Input: dimensioned drawing with shaded views. Units: mm. Origin: part minimum x, y, z. Give positions to 0.01 mm unless a question says otherwise; leave off trailing zeros. Loops run counter-clockwise (first coordinate to the right, second up) from the corner with the lowest first, then second, coordinate; pieces in that order, holes last.
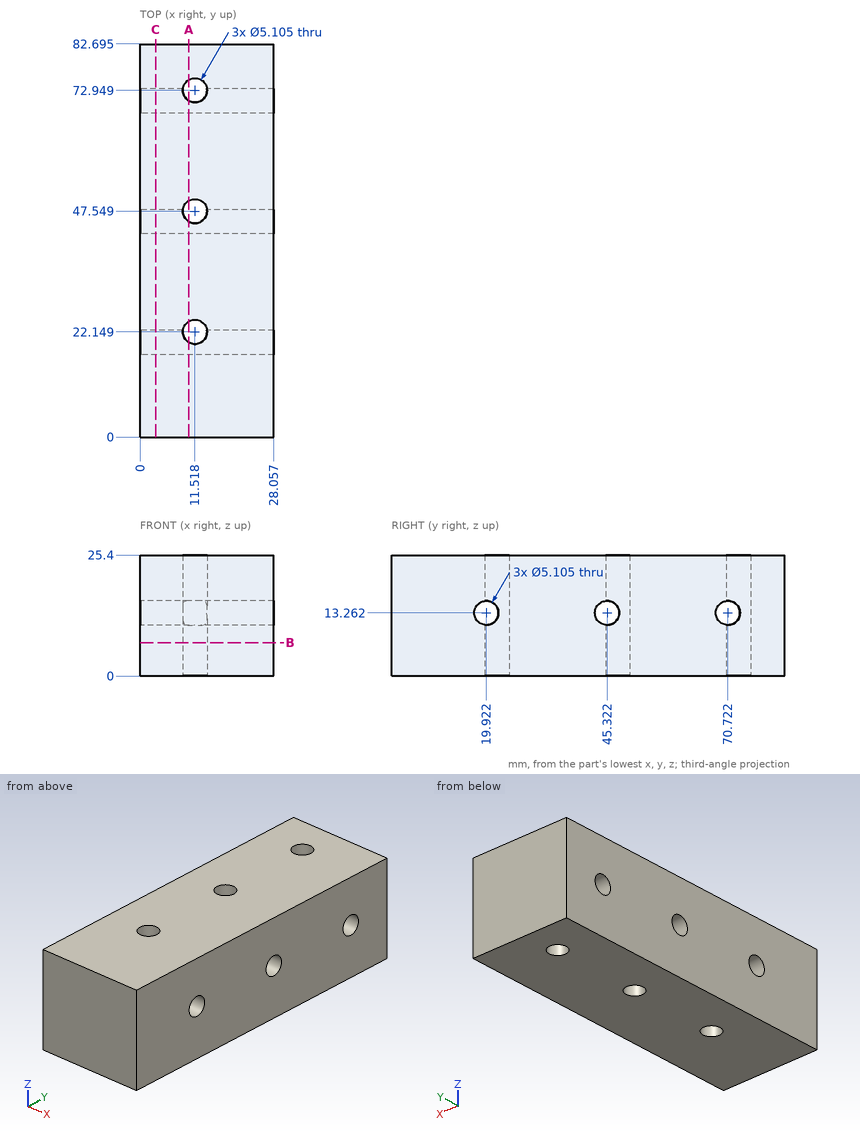
(1) Section C-C, the plane x = 3.25. Return the cut outline in (y, z) (1 decimal).
A:
outline: (0, 0) - (82.7, 0) - (82.7, 25.4) - (0, 25.4) - close; hole circle Ø5.1 at (19.9, 13.3); hole circle Ø5.1 at (45.3, 13.3); hole circle Ø5.1 at (70.7, 13.3)
(2) Section B-B, the plane z = 7. Return the cut outline in (x, y) (1 decimal), then the cut area to 3 significant figures.
A:
outline: (0, 0) - (28.1, 0) - (28.1, 82.7) - (0, 82.7) - close; hole circle Ø5.1 at (11.5, 22.1); hole circle Ø5.1 at (11.5, 47.5); hole circle Ø5.1 at (11.5, 72.9)
area: 2,260 mm2
(3) Ray query, line 1 along Y through (x, z) = (14.5, 13) (1 decimal); line 2 along Y through (x, z) = (4, 12.5) (1 decimal); line 3 along Z through (x, y) = (5, 71) (1 decimal). Return the intervals inside material, ascending.
A:
line 1: y = 0 to 17.4, 22.5 to 42.8, 47.9 to 68.2, 73.3 to 82.7
line 2: y = 0 to 17.5, 22.4 to 42.9, 47.8 to 68.3, 73.2 to 82.7
line 3: z = 0 to 10.7, 15.8 to 25.4
(4) First-contact query: pin 1 (8 mm diameter, centred on x = 11.52, y = 72.95, fed in from -Z). Flat tip, straight axial feed; report the tip coordinate or a pass-through.
A:
pin 1: stops at z = 0
(5) Section A-A, the plane x = 10.25. Return the cut outline in (y, z) (1 decimal), then the cut area to 3 significant figures.
A:
outline: (0, 0) - (19.9, 0) - (19.9, 10.7) arc R2.6 cw (long way) to (19.9, 15.8) - (19.9, 25.4) - (0, 25.4) - close; (24.4, 0) - (45.3, 0) - (45.3, 10.7) arc R2.6 cw (long way) to (45.3, 15.8) - (45.3, 25.4) - (24.4, 25.4) - close; (49.8, 0) - (70.7, 0) - (70.7, 10.7) arc R2.6 cw (long way) to (70.7, 15.8) - (70.7, 25.4) - (49.8, 25.4) - close; (75.2, 0) - (82.7, 0) - (82.7, 25.4) - (75.2, 25.4) - close
area: 1,730 mm2
